Geometry: final body of the model. Coordinates: model frame, mm. Face numbers are marked on the shaded views. A direction names the side the tool comes from. Round coordinates to 2 decimals unless told otherwise and drop trailing zeros. Loops run counter-clockwise (first coordinate to the right, second up) from the corner with the lowest first, then second, coordinate; pieces in that order, holes last. Notation, with made-up numbers: M 81,-14.75 L 110,-14.75 A5 cw 110,-8.75 Z; hole C -2.75,71.5 d7. An arc over 180 degrees is marked long. Answer as a JSON object with one key per item and string values.
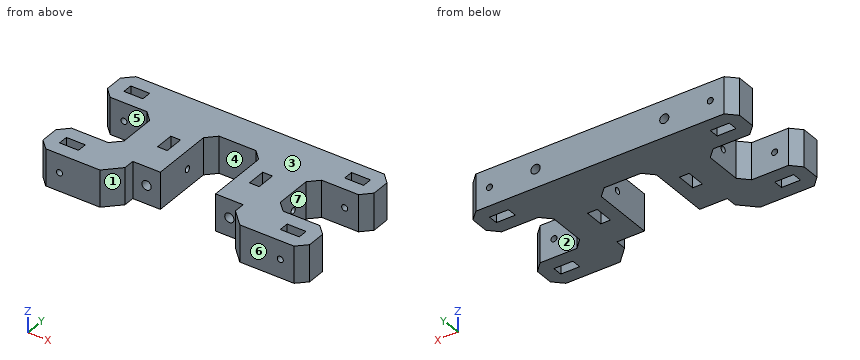
from build123d import *

# Parameters (mm, degrees)
SKETCH_1_W               = 10.3
SKETCH_1_H               = 5.3
SKETCH_1_W_2             = 5.3
SKETCH_1_H_2             = 10.3
EXTRUDE_2_DEPTH          = 20
CHAMFER_1_SIZE           = 5
CUT_EXTRUDE_1_REACH      = 104.744
SKETCH_2_R               = 1.65
CUT_EXTRUDE_2_REACH      = 123.861
SKETCH_4_R               = 1.65
MIRROR_2_COPY_1_REACH    = 104.744
MIRROR_2_COPY_1_SKETCH_R = 1.65
SKETCH_7_R               = 2.5
CUT_EXTRUDE_4_DEPTH      = 15
CUT_EXTRUDE_7_REACH      = 84.953
SKETCH_11_R              = 2.5
CUT_EXTRUDE_8_DEPTH      = 10


with BuildPart() as part:
    # 草圖1 → 填料-伸長2 (new body)
    with BuildSketch(Plane.XY):
        Polygon((15, 17.5), (15, -35), (72.5, -35), (72.5, -15), (42.5, -15), (42.5, 15), (72.5, 15), (72.5, 35), (-72.5, 35), (-72.5, 15), (-42.5, 15), (-42.5, -15), (-72.5, -15), (-72.5, -35), (-15, -35), (-15, 17.5), align=None)
        with Locations((-60, -25)):
            Rectangle(SKETCH_1_W, SKETCH_1_H, mode=Mode.SUBTRACT)
        with Locations((-60, 25)):
            Rectangle(SKETCH_1_W, SKETCH_1_H, mode=Mode.SUBTRACT)
        with Locations((-25, 0)):
            Rectangle(SKETCH_1_W_2, SKETCH_1_H_2, mode=Mode.SUBTRACT)
        with Locations((60, -25)):
            Rectangle(SKETCH_1_W, SKETCH_1_H, mode=Mode.SUBTRACT)
        with Locations((25, 0)):
            Rectangle(SKETCH_1_W_2, SKETCH_1_H_2, mode=Mode.SUBTRACT)
        with Locations((60, 25)):
            Rectangle(SKETCH_1_W, SKETCH_1_H, mode=Mode.SUBTRACT)
    extrude(amount=EXTRUDE_2_DEPTH)

    # 導角1
    chamfer_1_edges = [part.edges().sort_by_distance(p)[0] for p in [
        (-15, 17.5, 10),
        (-72.5, -35, 10),
        (-72.5, -15, 10),
        (-42.5, -15, 10),
        (-42.5, 15, 10),
        (-72.5, 15, 10),
        (-72.5, 35, 10),
        (72.5, 35, 10),
        (72.5, 15, 10),
        (42.5, 15, 10),
        (42.5, -15, 10),
        (72.5, -15, 10),
        (72.5, -35, 10),
        (15, 17.5, 10),
    ]]
    chamfer(chamfer_1_edges, length=CHAMFER_1_SIZE)

    # 除料-伸長1: up to this face of the body (flat: up to its plane)
    cut_extrude_1_end = Plane(part.part.faces().sort_by_distance((57.5, 15, 10))[0])
    # 草圖2 → 除料-伸長1 (cut, up to the picked face)
    with BuildSketch(Plane(origin=(0, 35, 0), x_dir=(1, 0, 0), z_dir=(0, 1, 0)), mode=Mode.PRIVATE) as cut_extrude_1_sk1:
        with Locations(Location((60, -10, 0), (0, 0, 270))):
            Circle(SKETCH_2_R)
    cut_extrude_1_tool1 = split(extrude(cut_extrude_1_sk1.sketch, amount=-CUT_EXTRUDE_1_REACH, mode=Mode.PRIVATE), bisect_by=cut_extrude_1_end, keep=Keep.BOTH, mode=Mode.PRIVATE)
    cut_extrude_1 = cut_extrude_1_tool1.solids().sort_by(Axis((60, 35, 10), (0, -1, 0)))[0]
    add(cut_extrude_1, mode=Mode.SUBTRACT)

    # 除料-伸長2: up to this face of the body (flat: up to its plane)
    cut_extrude_2_end = Plane(part.part.faces().sort_by_distance((15, -11.25, 10))[0])
    # 草圖4 → 除料-伸長2 (cut, up to the picked face)
    with BuildSketch(Plane(origin=(42.5, 0, 0), x_dir=(0, 0, -1), z_dir=(1, 0, 0)), mode=Mode.PRIVATE) as cut_extrude_2_sk1:
        with Locations((-10, 0)):
            Circle(SKETCH_4_R)
    cut_extrude_2_tool1 = split(extrude(cut_extrude_2_sk1.sketch, amount=-CUT_EXTRUDE_2_REACH, mode=Mode.PRIVATE), bisect_by=cut_extrude_2_end, keep=Keep.BOTH, mode=Mode.PRIVATE)
    cut_extrude_2 = cut_extrude_2_tool1.solids().sort_by(Axis((42.5, 0, 10), (-1, 0, 0)))[0]
    add(cut_extrude_2, mode=Mode.SUBTRACT)

    # 鏡射1: 除料-伸長1 across plane
    add(cut_extrude_1.mirror(Plane.ZX), mode=Mode.SUBTRACT)

    # 鏡射2: 除料-伸長1, 除料-伸長2 across plane
    add(cut_extrude_1.mirror(Plane(origin=(0, 0, 0), x_dir=(0, 0, 1), z_dir=(1, 0, 0))), mode=Mode.SUBTRACT)
    add(cut_extrude_2.mirror(Plane(origin=(0, 0, 0), x_dir=(0, 0, 1), z_dir=(1, 0, 0))), mode=Mode.SUBTRACT)

    # 鏡射2 copy 1: up to this face of the body (flat: up to its plane)
    mirror_2_copy_1_end = Plane(part.part.faces().sort_by_distance((-57.5, -15, 10))[0])
    # 鏡射2 copy 1 sketch → 鏡射2 copy 1 (cut, up to the picked face)
    with BuildSketch(Plane(origin=(0, -35, 0), x_dir=(-1, 0, 0), z_dir=(0, -1, 0)), mode=Mode.PRIVATE) as mirror_2_copy_1_sk1:
        with Locations(Location((60, -10, 0), (0, 0, 270))):
            Circle(MIRROR_2_COPY_1_SKETCH_R)
    mirror_2_copy_1_tool1 = split(extrude(mirror_2_copy_1_sk1.sketch, amount=-MIRROR_2_COPY_1_REACH, mode=Mode.PRIVATE), bisect_by=mirror_2_copy_1_end, keep=Keep.BOTH, mode=Mode.PRIVATE)
    add(mirror_2_copy_1_tool1.solids().sort_by(Axis((-60, -35, 10), (0, 1, 0)))[0], mode=Mode.SUBTRACT)

    # 草圖7 → 除料-伸長4 (cut)
    with BuildSketch(Plane(origin=(0, 35, 0), x_dir=(1, 0, 0), z_dir=(0, 1, 0))):
        with Locations(Location((35, -10, 0), (0, 0, 270))):
            Circle(SKETCH_7_R)
    cut_extrude_4 = extrude(amount=-CUT_EXTRUDE_4_DEPTH, mode=Mode.SUBTRACT)

    # 鏡射9: 除料-伸長4 across plane
    add(cut_extrude_4.mirror(Plane(origin=(0, 0, 0), x_dir=(0, 0, 1), z_dir=(1, 0, 0))), mode=Mode.SUBTRACT)

    # 草圖10 → 除料-伸長7 (cut, up to next)
    with BuildSketch(Plane.XY.offset(20), mode=Mode.PRIVATE) as cut_extrude_7_sk1:
        Polygon((15, -35), (15, -21), (30, -21), (30, -27), (38, -35), (30, -35), align=None)
    cut_extrude_7_tool1 = extrude(cut_extrude_7_sk1.sketch, amount=-CUT_EXTRUDE_7_REACH, mode=Mode.PRIVATE) & part.part
    cut_extrude_7 = cut_extrude_7_tool1.solids().sort_by_distance((23.844353, -28.573003, 20))[0]
    add(cut_extrude_7, mode=Mode.SUBTRACT)

    # 草圖11 → 除料-伸長8 (cut)
    with BuildSketch(Plane(origin=(0, -21, 0), x_dir=(-1, 0, 0), z_dir=(0, -1, 0))):
        with Locations(Location((-22.5, -10, 0), (0, 0, 90))):
            Circle(SKETCH_11_R)
    cut_extrude_8 = extrude(amount=-CUT_EXTRUDE_8_DEPTH, mode=Mode.SUBTRACT)

    # 鏡射10: 除料-伸長7, 除料-伸長8 across plane
    add(cut_extrude_7.mirror(Plane(origin=(0, 0, 0), x_dir=(0, 0, 1), z_dir=(1, 0, 0))), mode=Mode.SUBTRACT)
    add(cut_extrude_8.mirror(Plane(origin=(0, 0, 0), x_dir=(0, 0, 1), z_dir=(1, 0, 0))), mode=Mode.SUBTRACT)


solid = part.part
1) Reachability of the marked faces 4, 5, 6 and 7 from +Z, -Z, +X, -X, +Y, -Y: full face, straight path, thin tool, end or side. Return the list, or none.
Results:
{"face 4": "+Z, -Z, -Y", "face 5": "+Z, -Z, -X", "face 6": "+Z, -Z, +X, -X, -Y", "face 7": "+Z, -Z, +X"}
2) Section query B-B (x = -53). Return the cut outline in (y, z).
Results:
{"outline": "M -35,0 L -15,0 L -15,20 L -35,20 Z; M 15,0 L 35,0 L 35,20 L 15,20 Z"}
3) Section query A-A (y = -18). Return the cut outline in (x, z), and give its area (3 significant figures).
Results:
{"outline": "M -70.5,0 L -15,0 L -15,20 L -70.5,20 Z; M 15,0 L 70.5,0 L 70.5,20 L 15,20 Z; hole C -60,10 d3.3; hole C -22.5,10 d5; hole C 22.5,10 d5; hole C 60,10 d3.3", "area": "2,160 mm2"}
4) Ray query, line 1 (X direction, y = -25.5, z = 15.25); line 2 (Y direction, x = 57, z = 4.25); line 3 (Y direction, x = -51, z = 15.5). Return the intervals inside material, ascending.
Results:
{"line 1": "-72.5 to -65.15, -54.85 to -30, 30 to 54.85, 65.15 to 72.5", "line 2": "-35 to -27.65, -22.35 to -15, 15 to 22.35, 27.65 to 35", "line 3": "-35 to -15, 15 to 35"}
5) Pin query (flat end, axial travel): P1, Ø4, axis at y = 0, z = 10, coming from the +X side; P2, Ø6.5, axis at x = -35, z = 10, coming from the +Y side; P3, Ø2.5, axis at x = -34.5, z = 10, coming from the +Y side; P4, Ø11.5, axis at y = 1.5, z = 9.5, coming from the -X side. Return the tip coordinate at first contact, or that it passes through.
Results:
{"P1": "x = 42.5", "P2": "y = 35", "P3": "y = 20", "P4": "x = -42.5"}
6) Section query C-C (x = 60). Count the separate pieces of the cut face and the enclosed holes in it, and give its area (3 significant figures).
Results:
{"separate pieces": "8", "enclosed holes": "0", "area": "491 mm2"}
7) Pull-direction query (Y, two-part tool) for the marked faces 1, 2 and 3; classes: +Y half, -Y half, draft (parallel to the pull), parting line (faces both ways), or undercut.
Results:
{"face 1": "-Y half", "face 2": "undercut", "face 3": "draft"}
